```python
from build123d import *

# Parameters (mm, degrees)
SKETCH1_R           = 24.765
BOSS_EXTRUDE1_DEPTH = 2.286
SKETCH2_R           = 1.7145
CUT_EXTRUDE1_DEPTH  = 36.320159031
CUT_EXTRUDE2_DEPTH  = 36.320159031
CIRPATTERN1_COUNT   = 3
FILLET1_R           = 5
FILLET4_R           = 1
CHAMFER1_SIZE       = 0.5
CHAMFER2_SIZE       = 0.5
CHAMFER3_SIZE       = 0.25


with BuildPart() as part:
    # Sketch1 → Boss-Extrude1 (new, symmetric)
    with BuildSketch(Plane(origin=(0, 0, 0), x_dir=(1, 0, 0), z_dir=(0, 1, 0))):
        with Locations(Location((0, 0, 0), (0, 0, 270))):
            Circle(SKETCH1_R)
    extrude(amount=BOSS_EXTRUDE1_DEPTH, both=True)

    # Sketch2 → Cut-Revolve1 (revolve, cut)
    with BuildSketch(Plane(origin=(0, 0, 0), x_dir=(0, 0, -1), z_dir=(1, 0, 0))):
        with Locations((25.065, 0)):
            Circle(SKETCH2_R)
    revolve(axis=Axis((0, 0, 0), (0, 1, 0)), mode=Mode.SUBTRACT)

    # Sketch3 → Cut-Extrude1 (cut, through all)
    with BuildSketch(Plane(origin=(0, 2.286, 0), x_dir=(1, 0, 0), z_dir=(0, 1, 0))):
        with BuildLine():
            Line((1.372953022, 0.873), (-1.372953022, 0.873))
            ThreePointArc((-1.372953022, 0.873), (0, -1.627), (1.372953022, 0.873))
        make_face()
    extrude(amount=-CUT_EXTRUDE1_DEPTH, mode=Mode.SUBTRACT)

    # Sketch4 → Cut-Extrude2 (cut, through all)
    with BuildSketch(Plane(origin=(0, 2.286, 0), x_dir=(1, 0, 0), z_dir=(0, 1, 0))):
        with BuildLine():
            Line((3.742640687, 3.315515147), (17.462152397, 11.236478926))
            ThreePointArc((17.462152397, 11.236478926), (0, 20.765), (-17.462152397, 11.236478926))
            Line((-17.462152397, 11.236478926), (-3.742640687, 3.315515147))
            ThreePointArc((-3.742640687, 3.315515147), (0, 5), (3.742640687, 3.315515147))
        make_face()
    cut_extrude2 = extrude(amount=-CUT_EXTRUDE2_DEPTH, mode=Mode.SUBTRACT)

    # CirPattern1: Cut-Extrude2 ×3 about axis
    cirpattern1_axis = Axis((0, 0, 0), (0, 1, 0))
    for i in range(1, CIRPATTERN1_COUNT):
        add(cut_extrude2.rotate(cirpattern1_axis, i * 360 / CIRPATTERN1_COUNT), mode=Mode.SUBTRACT)

    # Fillet1
    fillet1_edges = [part.edges().sort_by_distance(p)[0] for p in [
        (3.742640687, 0, -3.315515147),
        (-3.742640687, 0, -3.315515147),
        (1, 0, 4.898979486),
        (4.742640687, 0, -1.583464339),
        (-4.742640687, 0, -1.583464339),
        (-1, 0, 4.898979486),
    ]]
    fillet(fillet1_edges, radius=FILLET1_R)

    # Fillet4
    fillet4_edges = [part.edges().sort_by_distance(p)[0] for p in [
        (-17.462152397, 0, -11.236478926),
        (17.462152397, 0, -11.236478926),
        (18.462152397, 0, -9.504428118),
        (1, 0, 20.740907044),
        (-1, 0, 20.740907044),
        (-18.462152397, 0, -9.504428118),
    ]]
    fillet(fillet4_edges, radius=FILLET4_R)

    # Chamfer1
    chamfer1_edges = [part.edges().sort_by_distance(p)[0] for p in [
        (0, -2.286, -0.873),
        (0, -2.286, 1.627),
        (0, 2.286, -0.873),
        (0, 2.286, 1.627),
    ]]
    chamfer(chamfer1_edges, length=CHAMFER1_SIZE)

    # Chamfer2
    chamfer2_edges = [part.edges().sort_by_distance(p)[0] for p in [
        (12.47866882, 2.286, -6.049862264),
        (12.47866882, -2.286, -6.049862264),
        (17.98301751, 2.286, 10.3825),
        (17.98301751, -2.286, 10.3825),
        (-17.98301751, 2.286, 10.3825),
        (-17.98301751, -2.286, 10.3825),
        (-11.47866882, 2.286, -7.781913072),
        (-11.47866882, -2.286, -7.781913072),
        (-1, 2.286, 13.831775336),
        (-1, -2.286, 13.831775336),
        (17.006931622, 2.286, -11.354272778),
        (17.006931622, -2.286, -11.354272778),
        (18.336554478, 2.286, -9.051298436),
        (18.336554478, -2.286, -9.051298436),
        (-18.336554478, 2.286, -9.051298436),
        (-18.336554478, -2.286, -9.051298436),
        (-17.006931622, 2.286, -11.354272778),
        (-17.006931622, -2.286, -11.354272778),
        (1.329622856, 2.286, 20.405571214),
        (1.329622856, -2.286, 20.405571214),
        (-1.329622856, 2.286, 20.405571214),
        (-1.329622856, -2.286, 20.405571214),
        (11.47866882, 2.286, -7.781913072),
        (11.47866882, -2.286, -7.781913072),
        (0, 2.286, -5),
        (0, -2.286, -5),
        (4.330127019, 2.286, 2.5),
        (4.330127019, -2.286, 2.5),
        (1, 2.286, 13.831775336),
        (1, -2.286, 13.831775336),
        (-4.330127019, 2.286, 2.5),
        (-4.330127019, -2.286, 2.5),
        (-12.47866882, 2.286, -6.049862264),
        (-12.47866882, -2.286, -6.049862264),
        (4.227779535, 2.286, -4.205135088),
        (4.227779535, -2.286, -4.205135088),
        (-4.227779535, 2.286, -4.205135088),
        (-4.227779535, -2.286, -4.205135088),
        (5.75564358, 2.286, -1.558796935),
        (5.75564358, -2.286, -1.558796935),
        (1.527864045, 2.286, 5.763932023),
        (1.527864045, -2.286, 5.763932023),
        (-1.527864045, 2.286, 5.763932023),
        (-1.527864045, -2.286, 5.763932023),
        (-5.75564358, 2.286, -1.558796935),
        (-5.75564358, -2.286, -1.558796935),
        (0, 2.286, -20.765),
        (0, -2.286, -20.765),
    ]]
    chamfer(chamfer2_edges, length=CHAMFER2_SIZE)

    # Chamfer3
    chamfer3_edges = [part.edges().sort_by_distance(p)[0] for p in [
        (0, -2.286, -24.765),
        (0, 2.286, -24.765),
    ]]
    chamfer(chamfer3_edges, length=CHAMFER3_SIZE)


solid = part.part
```
For this review, take the finished solid that the model builds, in its own axes (mm). A direction names the side the tool comes from. Coordinates: 2 decimals unless noted, no trailing zeros. Answer as CSV lines item,"result".
Q1. Clearance check with flat-ended pins moving along their axes: pin 1 Ø1.8 at (y, z) = (-0.5, 11.5) entering from +X; pin 2 Ø2 at (x, y) = (0.5, 0.5) entering from +Z; pin 3 Ø2 at (x, y) = (-3.5, 2) entering from +Z. State where each tip first meets the part, or that it passes through.
Model answer:
pin 1,"stops at x = 21.23"
pin 2,"stops at z = 24.23"
pin 3,"stops at z = 24.64"
Q2. For faces 1 (the face through (11.53, -2.03, -7.53)), 2 (the face through (-11.549, 0.025, -7.823)), 3 (the face through (-12.28, 2.04, -6.23)), list the 3-axis set-ups (+Z, -Z, +X, -X, +Y, -Y) from which the entire face can be reached by the end or side of a thin tool; tool diameter is ignored.
Model answer:
face 1,"-Y"
face 2,"+Y, -Y"
face 3,"+Y"
Q3. Wall thickness on line 1 along Z through (x, y) = (10.5, 0.55); line 2 along X through (y, z) = (0.75, 19); line 3 along X through (y, z) = (0.2, 0) (3 decimals): over which ranges is each line inside the solid? List them lowest first. Write a range as [from, to].
Model answer:
line 1,"z = [-20.96, -17.91], [-7.22, -4.91], [17.91, 20.96]"
line 2,"x = [-13.87, -8.38], [-1, 1], [8.38, 13.87]"
line 3,"x = [-23.362, -20.765], [-5.073, -1.627], [1.627, 5.073], [20.765, 23.362]"
Q4. We need section A-A (x = 11). Count the separate pieces of the cut face and the enclosed holes in it, plus the area to 3 significant figures.
Model answer:
separate pieces,"3"
enclosed holes,"0"
area,"43.0 mm2"
Q5. Draft analysis for pull direction X (two halves, no side actions). For faces 4 (the face through (7.44, 1.86, 23.62)), 5 (the face through (1, 0, 14)), state which applies: released by +X, released by -X, zero draft, split by the parting line, or undercut.
Model answer:
face 4,"split by the parting line"
face 5,"undercut"
